```python
from build123d import *

# Parameters (mm, degrees)
ESBO_O1_W                = 100
ESBO_O1_H                = 250
RESSALTO_EXTRUS_O1_DEPTH = 10
ESBO_O7_R                = 10
CORTE_EXTRUS_O6_DEPTH    = 9
ESBO_O2_W                = 28
ESBO_O2_H                = 26.8
RESSALTO_EXTRUS_O3_DEPTH = 25
ESBO_O8_W                = 2
ESBO_O8_H                = 12.8
CORTE_EXTRUS_O7_DEPTH    = 10
ESBO_O9_W                = 43
ESBO_O9_H                = 3
CORTE_EXTRUS_O8_DEPTH    = 2
ESBO_O10_W               = 100
ESBO_O10_H               = 46.5
CORTE_EXTRUS_O9_DEPTH    = 12
SKETCH1_R                = 2.5
CUT_EXTRUDE1_DEPTH       = 10


with BuildPart() as part:
    # Esboço1 → Ressalto-extrusão1 (new body)
    with BuildSketch(Plane.XY):
        with Locations((50, 125)):
            Rectangle(ESBO_O1_W, ESBO_O1_H)
    extrude(amount=RESSALTO_EXTRUS_O1_DEPTH)

    # Esboço7 → Corte-extrusão6 (cut)
    with BuildSketch(Plane.XY.offset(10)):
        with Locations((30, 98)):
            Circle(ESBO_O7_R)
        with Locations((30, 230)):
            Circle(ESBO_O7_R)
        with Locations(Location((70, 230, 0), (0, 0, 180))):
            Circle(ESBO_O7_R)
        with Locations(Location((70, 98, 0), (0, 0, 180))):
            Circle(ESBO_O7_R)
    extrude(amount=-CORTE_EXTRUS_O6_DEPTH, mode=Mode.SUBTRACT)

    # Esboço2 → Ressalto-extrusão3 (add)
    with BuildSketch(Plane.XY.offset(10)):
        with Locations((50, 68.4)):
            Rectangle(ESBO_O2_W, ESBO_O2_H)
        Polygon((50, 62), (43, 62), (43, 74.8), (57, 74.8), (57, 62), align=None, mode=Mode.SUBTRACT)
    extrude(amount=RESSALTO_EXTRUS_O3_DEPTH)

    # Esboço8 → Corte-extrusão7 (cut)
    with BuildSketch(Plane.XY.offset(10)):
        with Locations((44, 68.4)):
            Rectangle(ESBO_O8_W, ESBO_O8_H)
    extrude(amount=-CORTE_EXTRUS_O7_DEPTH, mode=Mode.SUBTRACT)

    # Esboço9 → Corte-extrusão8 (cut)
    with BuildSketch(Plane(origin=(0, 0, 0), x_dir=(-1, 0, 0), z_dir=(0, 0, -1))):
        with Locations((-21.5, 68.4)):
            Rectangle(ESBO_O9_W, ESBO_O9_H)
    extrude(amount=-CORTE_EXTRUS_O8_DEPTH, mode=Mode.SUBTRACT)

    # Esboço10 → Corte-extrusão9 (cut)
    with BuildSketch(Plane.XY.offset(10)):
        with Locations((50, 23.25)):
            Rectangle(ESBO_O10_W, ESBO_O10_H)
    extrude(amount=-CORTE_EXTRUS_O9_DEPTH, mode=Mode.SUBTRACT)

    # Sketch1 → Cut-Extrude1 (cut)
    with BuildSketch(Plane.XY.offset(10)):
        with Locations((6.5, 243.5)):
            Circle(SKETCH1_R)
        with Locations((93.5, 243.5)):
            Circle(SKETCH1_R)
        with Locations((6.5, 53)):
            Circle(SKETCH1_R)
        with Locations((93.5, 53)):
            Circle(SKETCH1_R)
    extrude(amount=-CUT_EXTRUDE1_DEPTH, mode=Mode.SUBTRACT)


solid = part.part
```
Check sheet for the modelled part. Datum: model origin and axes. Units: mm. A direction names the side the tool comes from. Give positions to 0.01 mm unless a question says otherwise; leave off trailing zeros. Write each loop counter-clockwise with the first axis right and the second up, starting at its lowest first coordinate (ties: lowest second). Pieces come first, ordered by that corner, then holes. Notation, with made-up numbers: (52, -1.75) -> (88, -1.75) arc R20 cw to (88, 5.25) -> close; hole circle Ø2 at (-11, 43.5). An arc over 180 degrees is marked (long way). Use CSV: the item, a comma, the result in double quotes. Start each with the question number.
Q1. Release check for a two-part mould opening along Y. For faces 5 (the flat face through (49, 250, 5)), 6 (the cylindrical face through (91, 53, 5)), 7 (the flat face through (50, 60, 35)) record: +Y half, -Y half, draft (parallel to the pull), parting line (faces both ways), or undercut.
Q2. Cross-section at A-A on y = 64.5. Enter the section's corners in (x, z), and give its area (3 significant figures).
Q3. Scan lines: line 1 along Y through (x, z) = (93.5, 6.75); line 2 along X through (y, z) = (243.5, 5); line 3 along Y through (x, z) = (30, 4). Record each from-to range of solid material in increasing order.
Q4. Tool access check on faces 1 (the flat face through (43, 68, 18)), 2 (the cylindrical face through (39.54, 233, 5.56)), 3 (the flat face through (36, 68, 22)), 4 (the flat face through (64, 68, 22)). Record the directions out of +Z, -Z, +X, -X, +Y, -Y that give a thin tool (end or side, any length) a straight path to the whole face; none if there is none.
Q5. Depth check by flat-ended pin: P1, Ø3, axis at y = 214, z = 12, coming from the -X side; P2, Ø12, axis at x = 30, y = 98, coming from the +Z side; P3, Ø1.5, axis at x = 47.5, y = 98.5, coming from the +Z side; P4, Ø10, axis at y = 69, z = 24, coming from the -X side. Enter the tip coordinate at first touch or a pass-through.
Q6. Cross-section at B-B on x = 93.5. Enter the section's corners in (y, z), and give its area (4 significant figures).
Q7. Cross-section at C-C on y = 243.5. Enter the section's corners in (x, z).
Q8. Cross-section at D-D on z = 22. Enter the section's corners in (x, y).
Working result:
1,face 5,"+Y half"
1,face 6,"undercut"
1,face 7,"draft"
2,outline,"(0, 0) -> (43, 0) -> (43, 35) -> (36, 35) -> (36, 10) -> (0, 10) -> close; (45, 0) -> (100, 0) -> (100, 10) -> (64, 10) -> (64, 35) -> (57, 35) -> (57, 10) -> (45, 10) -> close"
2,area,"1,330 mm^2"
3,line 1,"y = 46.5 to 50.5, 55.5 to 241, 246 to 250"
3,line 2,"x = 0 to 4, 9 to 91, 96 to 100"
3,line 3,"y = 46.5 to 88, 108 to 220, 240 to 250"
4,face 1,"+Z, -Z"
4,face 2,"+Z"
4,face 3,"+Z, -X, +Y, -Y"
4,face 4,"+Z, +X, +Y, -Y"
5,P1,"passes through"
5,P2,"stops at z = 1"
5,P3,"stops at z = 10"
5,P4,"stops at x = 36"
6,outline,"(46.5, 0) -> (50.5, 0) -> (50.5, 10) -> (46.5, 10) -> close; (55.5, 0) -> (241, 0) -> (241, 10) -> (55.5, 10) -> close; (246, 0) -> (250, 0) -> (250, 10) -> (246, 10) -> close"
6,area,"1,935 mm^2"
7,outline,"(0, 0) -> (4, 0) -> (4, 10) -> (0, 10) -> close; (9, 0) -> (91, 0) -> (91, 10) -> (9, 10) -> close; (96, 0) -> (100, 0) -> (100, 10) -> (96, 10) -> close"
8,outline,"(36, 55) -> (64, 55) -> (64, 81.8) -> (36, 81.8) -> close; hole (43, 62) -> (57, 62) -> (57, 74.8) -> (43, 74.8) -> close"
